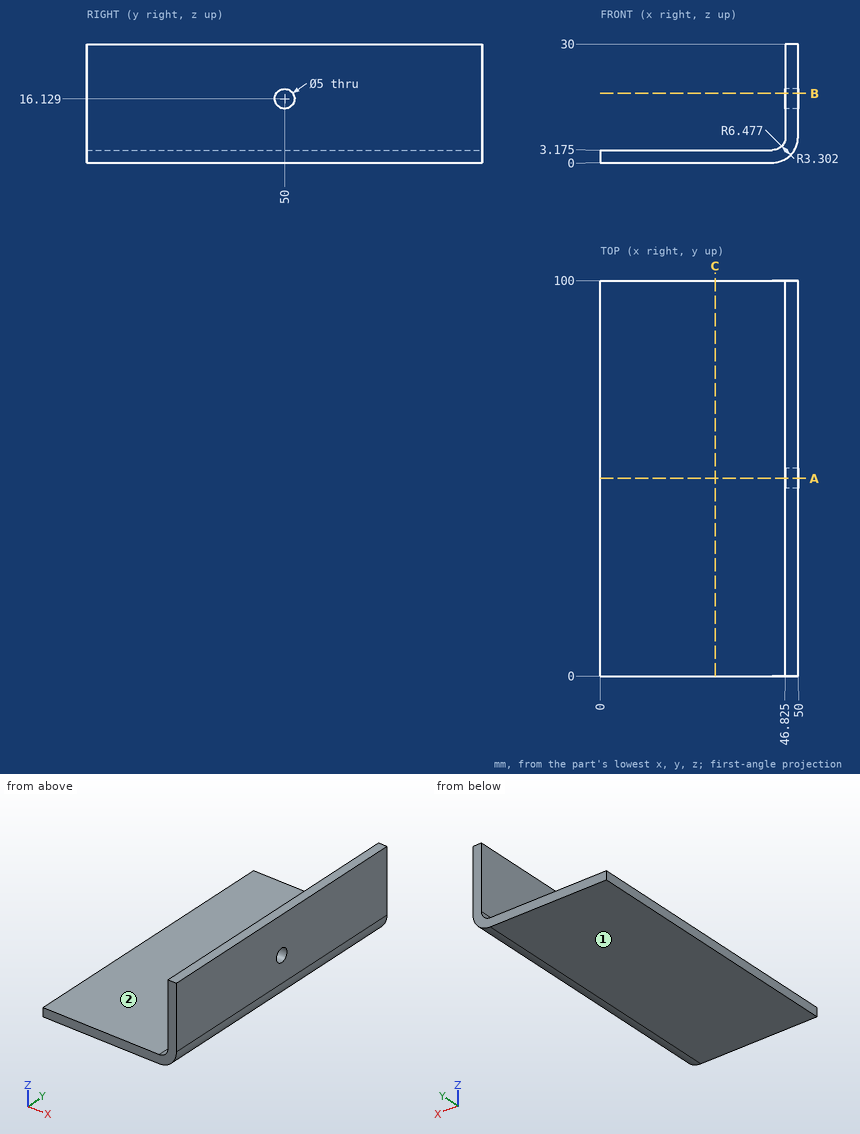
Study the drawing (mm; zero at the part's minimum x, y, z) and answer. A direction names the side the tool comes from. Give positions to 0.01 mm unless a question says otherwise; leave off trailing zeros. Order: outer loops, then holes, each group sorted by start corner. A loop starts at its lowest first (then second) coordinate and runs counter-clockwise, first axis right, second up. Notation, with made-up numbers: (-8.75, -13.5) -> (16.25, -13.5) arc R34 ccw to (16.25, 23.5) -> close; hole circle Ø9 at (74, 55.25). An arc over 180 degrees is marked (long way). Write item = value, one per line.
1. For the marked faces 1 and 2, determine the directions among +Z, -Z, +X, -X, +Y, -Y from which every point of the face is accessible in a straight line to the end or side of a thin tool.
Numbers:
face_1 = -Z, +X, -X, +Y, -Y
face_2 = +Z, -X, +Y, -Y
2. A cutting plane is placed at A-A, the plane y = 50. Write down the section's boundary in (x, z) (3 decimals).
Numbers:
outline = (0, 0) -> (43.523, 0) arc R6.477 ccw to (50, 6.477) -> (50, 13.629) -> (46.825, 13.629) -> (46.825, 6.477) arc R3.302 cw to (43.523, 3.175) -> (0, 3.175) -> close; (46.825, 18.629) -> (50, 18.629) -> (50, 30) -> (46.825, 30) -> close
3. Straight lines are drawn through the part: line 1 along X through (y, z) = (79, 16.25) (3 decimals); line 2 along Z through (x, y) = (42.5, 90) (3 decimals); line 3 along X through (y, z) = (81, 2). For each, find the intervals that lie inside material, in ascending order.
Numbers:
line_1 = 46.825 to 50
line_2 = 0 to 3.175
line_3 = 0 to 48.2
4. A cutting plane is placed at B-B, the plane z = 17.5. Write down the section's boundary in (x, y) (3 decimals), and give its area (3 significant figures).
Numbers:
outline = (46.825, 0) -> (50, 0) -> (50, 47.909) -> (46.825, 47.909) -> close; (46.825, 52.091) -> (50, 52.091) -> (50, 100) -> (46.825, 100) -> close
area = 304 mm²
5. A cutting plane is placed at C-C, the plane x = 29. Write down the section's boundary in (y, z) (3 decimals), and give its area (4 significant figures).
Numbers:
outline = (0, 0) -> (100, 0) -> (100, 3.175) -> (0, 3.175) -> close
area = 317.5 mm²
6. Given pin 1 (6 mm diameter, centred on x = 42.5, y = 37.5, fed in from +Z); pin 2 (12 mm diameter, centred on y = 57, z = 13, fed in from -X) (3 decimals); pin 3 (13 mm diameter, centred on x = 31, y = 55, fed in from +Z) (3 decimals), each flat-ended and moving along its own axis, determine where each tip first touches the part or whether it passes through.
Numbers:
pin_1 = 3.83
pin_2 = 46.825
pin_3 = 3.175
